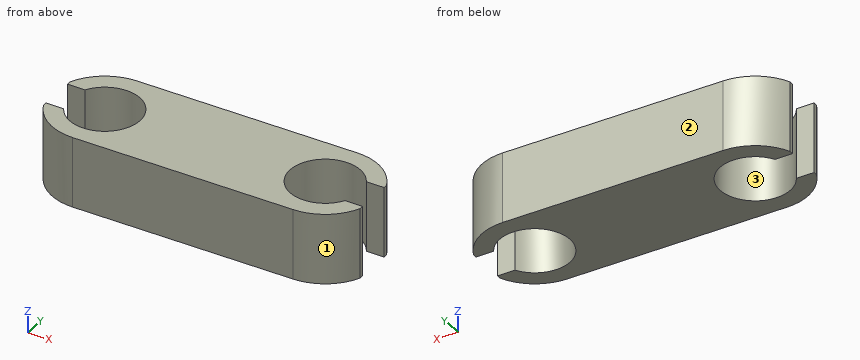
from build123d import *

# Parameters (mm, degrees)
SKETCH_1_R          = 1.5
EXTRUDE_1_DEPTH     = 2
CUT_EXTRUDE_1_DEPTH = 3


with BuildPart() as part:
    # 草图1 → 凸台-拉伸1 (new body)
    with BuildSketch(Plane.XY):
        with Locations((-3.13109105, 0)):
            Circle(SKETCH_1_R)
        with BuildLine():
            Line((3.13109105, 1.5), (-3.13109105, 1.5))
            ThreePointArc((-3.13109105, 1.5), (-2.070430878, 1.060660172), (-1.63109105, 0))
            ThreePointArc((-1.63109105, 0), (-2.070430878, -1.060660172), (-3.13109105, -1.5))
            Line((-3.13109105, -1.5), (3.13109105, -1.5))
            ThreePointArc((3.13109105, -1.5), (1.63109105, 0), (3.13109105, 1.5))
        make_face()
        with Locations((3.13109105, 0)):
            Circle(SKETCH_1_R)
    extrude(amount=EXTRUDE_1_DEPTH)

    # 草图2 → 切除-拉伸1 (cut)
    with BuildSketch(Plane.XY.offset(2)):
        with BuildLine():
            Line((-3.997116454, -0.5), (-4.497116454, -0.5))
            Line((-4.497116454, -0.5), (-4.497116454, -0.619656837))
            ThreePointArc((-4.497116454, -0.619656837), (-4.63109105, 0), (-4.497116454, 0.619656837))
            Line((-4.497116454, 0.619656837), (-4.497116454, 0.5))
            Line((-4.497116454, 0.5), (-3.997116454, 0.5))
            ThreePointArc((-3.997116454, 0.5), (-2.13109105, 0), (-3.997116454, -0.5))
        make_face()
        with BuildLine():
            Line((3.997116454, 0.5), (4.497116454, 0.5))
            Line((4.497116454, 0.5), (4.497116454, 0.619656837))
            ThreePointArc((4.497116454, 0.619656837), (4.63109105, 0), (4.497116454, -0.619656837))
            Line((4.497116454, -0.619656837), (4.497116454, -0.5))
            Line((4.497116454, -0.5), (3.997116454, -0.5))
            ThreePointArc((3.997116454, -0.5), (2.13109105, 0), (3.997116454, 0.5))
        make_face()
    extrude(amount=-CUT_EXTRUDE_1_DEPTH, mode=Mode.SUBTRACT)


solid = part.part
Source: CAD feature listing. Evaluate the final solid. Frame: model axes, mm. Face numbers are marked on the shaded views. Coordinates: 2 decimals unless noted, no trailing zeros. Loops run counter-clockwise (first coordinate to the right, second up) from the corner with the lowest first, then second, coordinate; pieces in that order, holes last. Notation, with made-up numbers: M -29.5,6.25 L -13.5,6.25 A13 cw -13.5,22.25 Z; hole C 2.5,-21 d4. An arc over 180 degrees is marked long. Answer in a Markdown table with one row per item.
Q1. Section C-C on z = 1. Return the cut outline in (x, y).
Answers below:
| item | result |
|---|---|
| outline | M -4.5,-0.62 A1.5 ccw -3.13,-1.5 L 3.13,-1.5 A1.5 ccw 4.5,-0.62 L 4.5,-0.5 L 4,-0.5 A1 cw long 4,0.5 L 4.5,0.5 L 4.5,0.62 A1.5 ccw 3.13,1.5 L -3.13,1.5 A1.5 ccw -4.5,0.62 L -4.5,0.5 L -4,0.5 A1 cw long -4,-0.5 L -4.5,-0.5 Z |
Q2. Section D-D on y = 0. Return the cut outline in (x, z), plus the area to 3 significant figures.
Answers below:
| item | result |
|---|---|
| outline | M -2.13,0 L 2.13,0 L 2.13,2 L -2.13,2 Z |
| area | 8.52 mm^2 |
Q3. Section A-A on x = 3. Return the cut outline in (y, z).
Answers below:
| item | result |
|---|---|
| outline | M -1.5,0 L -0.99,0 L -0.99,2 L -1.5,2 Z; M 0.99,0 L 1.5,0 L 1.5,2 L 0.99,2 Z |
Q4. First-contact query: pin 1 (1.6 mm diameter, centred on x = -3.13, y = 0, fed in from +Z). Flat tip, straight axial feed; report the tip coordinate or a pass-through.
Answers below:
| item | result |
|---|---|
| pin 1 | passes through |
Q5. Draft query along X for the marked faces 1, 2 and 3. Return one class per face: pulls with the +X half, pulls with the -X half, needs draft (parallel to the pull), parting line crosses it, or undercut.
Answers below:
| item | result |
|---|---|
| face 1 | pulls with the +X half |
| face 2 | needs draft |
| face 3 | undercut |
Q6. Section B-B on y = -0.9. Return the cut outline in (x, z).
Answers below:
| item | result |
|---|---|
| outline | M -4.33,0 L -3.57,0 L -3.57,2 L -4.33,2 Z; M -2.7,0 L 2.7,0 L 2.7,2 L -2.7,2 Z; M 3.57,0 L 4.33,0 L 4.33,2 L 3.57,2 Z |
Q7. Ray query, probe 1 along Y at (x, z) = (4.25, 0.2); probe 2 along X at (y, z) = (0.55, 0.1); probe 3 along X at (y, z) = (0, 0.95). Return the intervals inside material, ascending. Write a range as from..to.
Answers below:
| item | result |
|---|---|
| probe 1 | y = -1..-0.5, 0.5..1 |
| probe 2 | x = -4.5..-3.97, -2.3..2.3, 3.97..4.5 |
| probe 3 | x = -2.13..2.13 |
